For this review, take the finished solid that the model builds, in its own axes (mm). Face numbers are marked on the shaded views. A direction names the side the tool comes from. Coordinates: 2 decimals unless noted, no trailing zeros. Write each loop counter-clockwise with the first axis right and the second up, starting at its lowest first coordinate (ties: lowest second). Pieces come first, ordered by that corner, then holes. Notation, with made-up numbers: (-1.5, 62) - (55.5, 62) arc R29 cw to (55.5, 93) - close; hole circle Ø2 at (10.5, 60.5). An arc over 180 degrees is marked (long way). Write each question's results on one line, items separated by ' | '.
from build123d import *

# Parameters (mm, degrees)
SKETCH1_R           = 30
BASE_DEPTH          = 20
BOSS_EXTRUDE1_DEPTH = 20
CUT_EXTRUDE1_DEPTH  = 37
CIRPATTERN1_COUNT   = 4
BOSS_EXTRUDE2_START = 20
SKETCH1_10_R        = 15
BOSS_EXTRUDE2_DEPTH = 10
BOSS_EXTRUDE2_TAPER = 10
SKETCH1_11_R        = 6.5
CUT_EXTRUDE2_DEPTH  = 31.0000001
SKETCH1_12_W        = 4
SKETCH1_12_H        = 4
BOSS_EXTRUDE3_DEPTH = 25


with BuildPart() as part:
    # Sketch1 → Base (new body)
    with BuildSketch(Plane(origin=(0, 0, 0), x_dir=(1, 0, 0), z_dir=(0, 1, 0))):
        with Locations(Location((0, 0, 0), (0, 0, 270))):  # turned: the seam where the file's is
            Circle(SKETCH1_R)
    extrude(amount=BASE_DEPTH)

    # Sketch1_8 → Boss-Extrude1 (add)
    with BuildSketch(Plane(origin=(0, 0, 0), x_dir=(1, 0, 0), z_dir=(0, 1, 0))):
        with BuildLine():
            ThreePointArc((6, -29.393876913), (0, -30), (-6, -29.393876913))
            Line((-6, -29.393876913), (-6, -94.393876913))
            Line((-6, -94.393876913), (6, -94.393876913))
            Line((6, -94.393876913), (6, -29.393876913))
        make_face()
    boss_extrude1 = extrude(amount=BOSS_EXTRUDE1_DEPTH)

    # Sketch2 → Cut-Extrude1 (cut, through all)
    with BuildSketch(Plane.ZY.offset(6)):
        Polygon((29.393876913, 20), (94.393876913, 20), (94.393876913, 6.602540378), (79.393876913, 6.602540378), align=None)
    cut_extrude1 = extrude(amount=-CUT_EXTRUDE1_DEPTH, mode=Mode.SUBTRACT)

    # CirPattern1: Boss-Extrude1, Cut-Extrude1 ×4 about axis
    cirpattern1_axis = Axis((0, 0, 0), (0, 1, 0))
    add([boss_extrude1.rotate(cirpattern1_axis, i * 360 / CIRPATTERN1_COUNT) for i in range(1, CIRPATTERN1_COUNT)])
    add([cut_extrude1.rotate(cirpattern1_axis, i * 360 / CIRPATTERN1_COUNT) for i in range(1, CIRPATTERN1_COUNT)], mode=Mode.SUBTRACT)

    # Sketch1_10 → Boss-Extrude2 (add)
    with BuildSketch(Plane(origin=(0, 0, 0), x_dir=(1, 0, 0), z_dir=(0, 1, 0)).offset(BOSS_EXTRUDE2_START)):
        Circle(SKETCH1_10_R)
    extrude(amount=BOSS_EXTRUDE2_DEPTH, taper=BOSS_EXTRUDE2_TAPER)

    # Sketch1_11 → Cut-Extrude2 (cut, through all)
    with BuildSketch(Plane(origin=(0, 0, 0), x_dir=(1, 0, 0), z_dir=(0, 1, 0))):
        with Locations(Location((0, 0, 0), (0, 0, 270))):  # turned: the seam where the file's is
            Circle(SKETCH1_11_R)
    extrude(amount=CUT_EXTRUDE2_DEPTH, mode=Mode.SUBTRACT)

    # Sketch1_12 → Boss-Extrude3 (add)
    with BuildSketch(Plane(origin=(0, 0, 0), x_dir=(1, 0, 0), z_dir=(0, 1, 0))):
        with Locations((0, -26)):
            Rectangle(SKETCH1_12_W, SKETCH1_12_H)
    extrude(amount=BOSS_EXTRUDE3_DEPTH)


solid = part.part
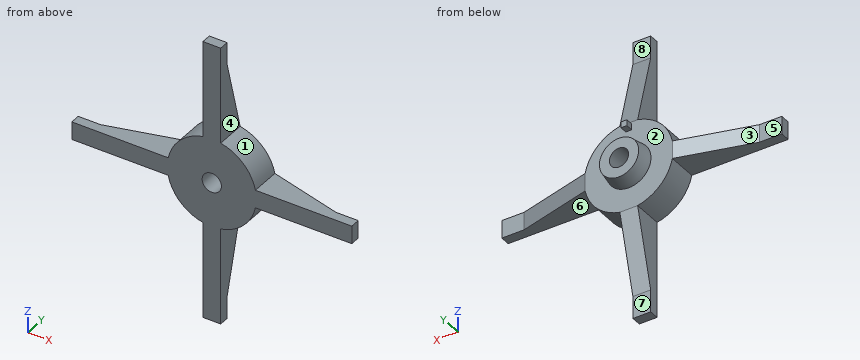
Q1. Take a section at D-D on x = -59.5. State the section outline as (y, z) points.
Results found:
outline: (0, -6) - (11.93, -6) - (11.93, 6) - (0, 6) - close
Q2. Take a section at B-B on z = -82. State the section outline as (x, y) points, plus the area to 3 significant figures.
Results found:
outline: (-6, 0) - (6, 0) - (6, 6.6) - (-6, 6.6) - close | area: 79.2 mm2
Q3. Mouldability with a two-part tool opening along X and no side actions: class the marked faces 1, 2 and 3 as pulls with the +X half, pulls with the -X half, needs draft (parallel to the pull), parting line crosses it, or undercut.
Results found:
face 1: pulls with the +X half | face 2: needs draft | face 3: pulls with the -X half
Q4. For the marked faces 4, 5, 6, 7 and 8, list the 3-axis set-ups (+Z, -Z, +X, -X, +Y, -Y) from which the entire face can be reached by the end or side of a thin tool; tool diameter is ignored.
Results found:
face 4: +Z, +X, +Y, -Y | face 5: +Z, -Z, -X, +Y | face 6: -Z, +X, +Y, -Y | face 7: -Z, +X, -X, +Y | face 8: +Z, +X, -X, +Y
Q5. Wall thickness on line 1 along Z through (x, y) = (-57.5, 2); line 2 along Y through (x, z) = (18, 4); line 3 along Z through (x, y) = (5, 21): over which ranges is each line inside the solid? List them lowest first. Write a range as from..to.
Results found:
line 1: -6..6 | line 2: 0..20 | line 3: -13.95..-4.15, 4.15..13.95
Q6. Take a section at A-A on y = 3. State the section outline as (x, z) points.
Results found:
outline: (-94.39, -6) - (-29.39, -6) arc R30 ccw to (-6, -29.39) - (-6, -94.39) - (6, -94.39) - (6, -29.39) arc R30 ccw to (29.39, -6) - (94.39, -6) - (94.39, 6) - (29.39, 6) arc R30 ccw to (6, 29.39) - (6, 94.39) - (-6, 94.39) - (-6, 29.39) arc R30 ccw to (-29.39, 6) - (-94.39, 6) - close; hole circle Ø13 at (0, 0)
Q7. For pin 1 (8 mm diameter, centred on y = 9, z = -73, fed in from +X); pin 2 (4 mm diameter, centred on x = -68, y = 3.5, fed in from +Z); pin 3 (1.2 mm diameter, centred on x = 0.5, z = 25.5, fed in from +Y); pin 4 (17 mm diameter, centred on x = 0, z = 0, fed in from +Y), all flat-tipped, find the tip position at first contact; note any pin that passes through.
Results found:
pin 1: x = 6 | pin 2: z = 6 | pin 3: y = 25 | pin 4: y = 30
Q8. Take a section at C-C on y = 17.5. State the section outline as (x, z) points.
Results found:
outline: (-38.72, -6) - (-29.39, -6) arc R30 ccw to (-6, -29.39) - (-6, -38.72) - (6, -38.72) - (6, -29.39) arc R30 ccw to (29.39, -6) - (38.72, -6) - (38.72, 6) - (29.39, 6) arc R30 ccw to (6, 29.39) - (6, 38.72) - (-6, 38.72) - (-6, 29.39) arc R30 ccw to (-29.39, 6) - (-38.72, 6) - close; hole circle Ø13 at (0, 0)
